Input: part model. Units: mm. Frame: model coordinates. A direction names the side the tool comes from. Round coordinates to 2 decimals unless told otherwise and drop trailing zeros. Return JSON: item names as keys, results as strings. Group by question number.
1) Material intervals for line 1 (X direction, y = 4.5, z = 1.3); line 2 (X direction, y = 3.25, z = 4.5); line 3 (Y direction, x = 0, z = 4.4), sorted ascending. Write a range as from..to.
2) Mould query, pull axis X, two halves, no side actions, for faces 1 (the face through (-0.54, -2.44, 4.02)), 2 (the face through (0, 2, 0)). Classes: +X half, -X half, draft (parallel to the pull), parting line (faces both ways), or undercut.
3) Contact query for a flat-ended pin moving along its axis: P1, Ø1.5, axis at x = 5, y = -3, coming from the +Z side. Output: stop coordinate, or through.
4) Access query for faces 3 (the face through (2, -1, 3.263)), 4 (the face through (-6.643, 4.748, 1.707)). Directions: +Z, -Z, +X, -X, +Y, -Y. A direction counts if a zero-diameter tool reaches every point of the face in a straight line with its end or side. Return the directions, or none.
5) Section A-A (x = -4.75). Count the separate pieces of the cut face and the enclosed holes in it, plus the area to 3 significant figures.
from build123d import *

# Parameters (mm, degrees)
BOSS_EXTRUDE1_DEPTH                               = 4.763
CSK_FOR_M2_5_FLAT_HEAD_MACHINE_SCREW1_D           = 2.9
CSK_FOR_M2_5_FLAT_HEAD_MACHINE_SCREW1_CSINK_D     = 5.5
CSK_FOR_M2_5_FLAT_HEAD_MACHINE_SCREW1_CSINK_ANGLE = 90
TAP_DRILL_FOR_M4X0_7_TAP1_D                       = 3.3
SKETCH8_R                                         = 2.5
CUT_EXTRUDE1_DEPTH                                = 1.5


with BuildPart() as part:
    # Sketch1 → Boss-Extrude1 (new body)
    with BuildSketch(Plane.XY):
        with BuildLine():
            ThreePointArc((-8.131727984, 2.474873734), (-8.131727984, 8.131727984), (-2.474873734, 8.131727984))
            add(Edge.make_bspline(
                [(-2.474873734, 8.131727984), (0, 3.868272016), (2.474873734, 8.131727984)],
                knots=[0, 0, 0, 1, 1, 1], degree=2))
            ThreePointArc((2.474873734, 8.131727984), (8.131727984, 8.131727984), (8.131727984, 2.474873734))
            add(Edge.make_bspline(
                [(8.131727984, 2.474873734), (3.868272016, 0), (8.131727984, -2.474873734)],
                knots=[0, 0, 0, 1, 1, 1], degree=2))
            ThreePointArc((8.131727984, -2.474873734), (8.131727984, -8.131727984), (2.474873734, -8.131727984))
            add(Edge.make_bspline(
                [(2.474873734, -8.131727984), (0, -3.868272016), (-2.474873734, -8.131727984)],
                knots=[0, 0, 0, 1, 1, 1], degree=2))
            ThreePointArc((-2.474873734, -8.131727984), (-8.131727984, -8.131727984), (-8.131727984, -2.474873734))
            add(Edge.make_bspline(
                [(-8.131727984, -2.474873734), (-3.868272016, 0), (-8.131727984, 2.474873734)],
                knots=[0, 0, 0, 1, 1, 1], degree=2))
        make_face()
    extrude(amount=BOSS_EXTRUDE1_DEPTH)

    # CSK for M2.5 Flat Head Machine Screw1 (through all)
    with Locations(Plane.XY.offset(4.763)):
        with Locations((-5.303300859, 5.303300859), (5.303300859, 5.303300859), (5.303300859, -5.303300859), (-5.303300859, -5.303300859)):
            CounterSinkHole(CSK_FOR_M2_5_FLAT_HEAD_MACHINE_SCREW1_D / 2, CSK_FOR_M2_5_FLAT_HEAD_MACHINE_SCREW1_CSINK_D / 2, counter_sink_angle=CSK_FOR_M2_5_FLAT_HEAD_MACHINE_SCREW1_CSINK_ANGLE)

    # Tap Drill for M4x0.7 Tap1 (through all)
    with Locations(Plane.XY.offset(4.763)):
        with Locations((0, 0)):
            Hole(TAP_DRILL_FOR_M4X0_7_TAP1_D / 2)

    # Sketch8 → Cut-Extrude1 (cut)
    with BuildSketch(Plane.XY.offset(4.763)):
        Circle(SKETCH8_R)
    extrude(amount=-CUT_EXTRUDE1_DEPTH, mode=Mode.SUBTRACT)


solid = part.part
Returned:
{
 "1": {"line 1": "x = -9.22..-6.51, -4.1..4.1, 6.51..9.22", "line 2": "x = -8.74..-6.71, -3.9..3.9, 6.71..8.74", "line 3": "y = -6..-2.5, 2.5..6"},
 "2": {"face 1": "undercut", "face 2": "draft"},
 "3": {"P1": "stops at z = 4.76"},
 "4": {"face 3": "+Z", "face 4": "+Z, -Z"},
 "5": {"separate pieces": "3", "enclosed holes": "0", "area": "59.2 mm^2"}
}
